```python
from build123d import *

# Parameters (mm, degrees)
BOSS_EXTRUDE1_DEPTH = 6
SKETCH2_R           = 2
CUT_EXTRUDE1_DEPTH  = 6
SKETCH3_R           = 5.75
SKETCH3_R_2         = 1.5
BOSS_EXTRUDE2_DEPTH = 12


with BuildPart() as part:
    # Sketch1 → Boss-Extrude1 (new body)
    with BuildSketch(Plane(origin=(0, 0, 0), x_dir=(0, 0, -1), z_dir=(1, 0, 0))):
        Polygon((3.393898061, -6.039988075), (6.927732142, -0.080792099), (3.533834081, 5.959195977), (-3.393898061, 6.039988075), (-6.927732142, 0.080792099), (-3.533834081, -5.959195977), align=None)
    extrude(amount=BOSS_EXTRUDE1_DEPTH)

    # Sketch2 → Cut-Extrude1 (cut)
    with BuildSketch(Plane(origin=(6, 0, 0), x_dir=(0, 0, -1), z_dir=(1, 0, 0))):
        Circle(SKETCH2_R)
    extrude(amount=-CUT_EXTRUDE1_DEPTH, mode=Mode.SUBTRACT)

    # Sketch3 → Boss-Extrude2 (add)
    with BuildSketch(Plane(origin=(6, 0, 0), x_dir=(0, 0, -1), z_dir=(1, 0, 0))):
        Circle(SKETCH3_R)
        Circle(SKETCH3_R_2, mode=Mode.SUBTRACT)
    extrude(amount=BOSS_EXTRUDE2_DEPTH)


solid = part.part
```
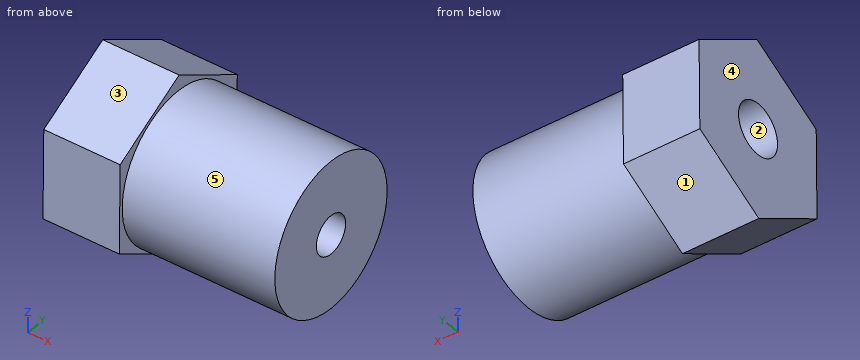
The listing builds one solid part. Answer for the finished solid, in the listing's coordinates (mm). Face numbers are marked on the shaded views. A direction names the side the tool comes from. Coordinates: 2 decimals unless noted, no trailing zeros. Loops run counter-clockwise (first coordinate to the right, second up) from the corner with the lowest first, then second, coordinate; pieces in that order, holes last. Notation, with made-up numbers: (-24.75, 59) - (33.25, 59) arc R15 cw to (33.25, 81) - close; hole circle Ø10 at (1.25, 84). An arc over 180 degrees is marked (long way). Use a Markdown table: item, result. Add a question column.
1) The part is cut by section D-D, the plane z = -1.75. Give the vertices of the cut face in (x, y), and give its area (3 significant figures).
2) The part is cut by section C-C, the plane x = 7. Give the vertices of the cut face in (y, z).
3) For the marked faces 4 and 5, determine the directions among +Z, -Z, +X, -X, +Y, -Y from which every point of the face is accessible in a straight line to the end or side of a thin tool.
4) The mould has two halves that part along Z. Classify the marked faces 1, 2 and 3: released by +Z, released by -Z, zero draft, split by the parting line, or undercut.
5) Given pin 1 (6 mm diameter, centred on x = 13, z = 0, fed in from +Y); pin 2 (6 mm diameter, centred on y = 2.5, z = 3, fed in from -X); pin 3 (1.5 mm diameter, centred on x = 14.5, y = -3, fed in from -Z); pin 4 (4 mm diameter, centred on x = 11.5, z = -5.5, fed in from +Y), each flat-ended and moving along its own axis, determine where each tip first touches the part or whether it passes through.
6) The part is cut by section A-A, the plane z = 0. Give the vertices of the cut face in (x, y).
7) Find the intervals of material crossed by line 1 (Y direction, x = 11.5, z = 0); line 2 (X direction, y = -2, z = -5.75); line 3 (Y direction, x = 4.6, z = 0), in increasing order.
8) The part is cut by section B-B, the plane y = 1. Give the vertices of the cut face in (x, z), and give its area (3 significant figures).
Here are the results:
| question | item | result |
|---|---|---|
| 1 | outline | (0, -6.02) - (6, -6.02) - (6, -5.48) - (18, -5.48) - (18, 5.48) - (6, 5.48) - (6, 5.98) - (0, 5.98) - (0, 0.97) - (6, 0.97) - (6, -0.97) - (0, -0.97) - close |
| 1 | area | 192 mm^2 |
| 2 | outline | circle Ø11.5 at (0, 0); hole circle Ø3 at (0, 0) |
| 3 | face 4 | +Z, -Z, -X, +Y, -Y |
| 3 | face 5 | +X |
| 4 | face 1 | released by -Z |
| 4 | face 2 | undercut |
| 4 | face 3 | released by +Z |
| 5 | pin 1 | stops at y = 5.75 |
| 5 | pin 2 | stops at x = 0 |
| 5 | pin 3 | stops at z = -5.29 |
| 5 | pin 4 | stops at y = 4.56 |
| 6 | outline | (0, -6) - (6, -6) - (6, -5.75) - (18, -5.75) - (18, -1.5) - (6, -1.5) - (6, -2) - (0, -2) - close; (0, 2) - (6, 2) - (6, 1.5) - (18, 1.5) - (18, 5.75) - (6, 5.75) - (6, 6) - (0, 6) - close |
| 7 | line 1 | y = -5.75 to -1.5, 1.5 to 5.75 |
| 7 | line 2 | x = 0 to 6 |
| 7 | line 3 | y = -6 to -2, 2 to 6 |
| 8 | outline | (0, -6.32) - (6, -6.32) - (6, -5.66) - (18, -5.66) - (18, -1.12) - (6, -1.12) - (6, -1.73) - (0, -1.73) - close; (0, 1.73) - (6, 1.73) - (6, 1.12) - (18, 1.12) - (18, 5.66) - (6, 5.66) - (6, 6.38) - (0, 6.38) - close |
| 8 | area | 164 mm^2 |
